Read the model definition and answer for the solid it produces. Units are mm, in the model's axes. A direction names the side the tool comes from. Round coordinates to 2 decimals unless told otherwise and drop trailing zeros. Loops run counter-clockwise (first coordinate to the right, second up) from the corner with the lowest first, then second, coordinate; pieces in that order, holes last. Notation, with made-up numbers: (72, 17) - (124, 17) arc R37 cw to (124, 53) - close; hole circle Ø2 at (62.25, 42). An arc over 180 degrees is marked (long way). Answer as CSV lines item,"result".
```python
from build123d import *

# Parameters (mm, degrees)
F0_W     = 74.8
F0_H     = 134.8
F0_W_2   = 3.605619
F0_H_2   = 110.626959
F1_DEPTH = 4


with BuildPart() as f1:
    # F0 (on Top) → F1 (new body)
    with BuildSketch(Plane.XY):
        Rectangle(F0_W, F0_H)
        with Locations((-30.278574, -0.018355)):
            Rectangle(F0_W_2, F0_H_2, mode=Mode.SUBTRACT)
        with Locations((-15.078575, -0.018355)):
            Rectangle(F0_W_2, F0_H_2, mode=Mode.SUBTRACT)
        with Locations((0.121425, -0.018355)):
            Rectangle(F0_W_2, F0_H_2, mode=Mode.SUBTRACT)
        with Locations((15.321426, -0.018355)):
            Rectangle(F0_W_2, F0_H_2, mode=Mode.SUBTRACT)
        with Locations((30.521425, -0.018355)):
            Rectangle(F0_W_2, F0_H_2, mode=Mode.SUBTRACT)
    extrude(amount=F1_DEPTH)


solid = f1.part
```
1) A cutting plane is placed at B-B, the plane z = 3.2. Determine the outline of the cut face in (x, y), plus the area to 3 significant figures.
Entries:
outline,"(-37.4, -67.4) - (37.4, -67.4) - (37.4, 67.4) - (-37.4, 67.4) - close; hole (-32.08, -55.33) - (-28.48, -55.33) - (-28.48, 55.3) - (-32.08, 55.3) - close; hole (-16.88, -55.33) - (-13.28, -55.33) - (-13.28, 55.3) - (-16.88, 55.3) - close; hole (-1.68, -55.33) - (1.92, -55.33) - (1.92, 55.3) - (-1.68, 55.3) - close; hole (13.52, -55.33) - (17.12, -55.33) - (17.12, 55.3) - (13.52, 55.3) - close; hole (28.72, -55.33) - (32.32, -55.33) - (32.32, 55.3) - (28.72, 55.3) - close"
area,"8,090 mm^2"
2) A cutting plane is placed at A-A, the plane y = -42.5. Determine the outline of the cut face in (x, z), plus the area to 3 significant figures.
Entries:
outline,"(-37.4, 0) - (-32.08, 0) - (-32.08, 4) - (-37.4, 4) - close; (-28.48, 0) - (-16.88, 0) - (-16.88, 4) - (-28.48, 4) - close; (-13.28, 0) - (-1.68, 0) - (-1.68, 4) - (-13.28, 4) - close; (1.92, 0) - (13.52, 0) - (13.52, 4) - (1.92, 4) - close; (17.12, 0) - (28.72, 0) - (28.72, 4) - (17.12, 4) - close; (32.32, 0) - (37.4, 0) - (37.4, 4) - (32.32, 4) - close"
area,"227 mm^2"
3) The mould has two halves that part along X. Classify faces 1 (the face through (-9, 1, 0)), 2 (the face through (37.4, -1, 2)), 3 (the face through (15, 55.295, 2)): pulls with the +X half, pulls with the -X half, needs draft (parallel to the pull), parting line crosses it, or undercut.
Entries:
face 1,"needs draft"
face 2,"pulls with the +X half"
face 3,"undercut"
4) A tool of negligible diameter and unlimited length cuts with its end or side. For faces 4 (the face through (-9, 1, 4)), 5 (the face through (0, -55.332, 2)), from which of +Z, -Z, +X, -X, +Y, -Y can it reach the whole face along a straight path? Write none if from no direction.
Entries:
face 4,"+Z, +X, -X, +Y, -Y"
face 5,"+Z, -Z"
5) Find the intervals of material crossed by line 1 (X direction, y = -9.5, z = 0.4); line 2 (Y direction, x = -30, z = 3.35), in increasing order.
Entries:
line 1,"x = -37.4 to -32.08, -28.48 to -16.88, -13.28 to -1.68, 1.92 to 13.52, 17.12 to 28.72, 32.32 to 37.4"
line 2,"y = -67.4 to -55.33, 55.3 to 67.4"
